from build123d import *

# Parameters (mm, degrees)
F0_R     = 23
F0_R_2   = 20
F1_DEPTH = 20
F2_R     = 23
F3_DEPTH = 5
F4_R     = 1
F5_R     = 1


with BuildPart() as f1:
    # F0 (on Top) → F1 (new body)
    with BuildSketch(Plane.XY):
        Circle(F0_R)
        Circle(F0_R_2, mode=Mode.SUBTRACT)
    extrude(amount=F1_DEPTH)

    # F2 (on face) → F3 (join)
    with BuildSketch(Plane.XY.offset(20)):
        Circle(F2_R)
    extrude(amount=F3_DEPTH)

    # F4
    f4_edges = [f1.edges().sort_by_distance(p)[0] for p in [
        (-20, 0, 0),
    ]]
    fillet(f4_edges, radius=F4_R)

    # F5
    f5_edges = [f1.edges().sort_by_distance(p)[0] for p in [
        (-23, 0, 0),
    ]]
    fillet(f5_edges, radius=F5_R)


solid = f1.part
Here's how the part is built. I have some questions about the finished solid (model axes, mm). Round coordinates to 2 decimals unless told otherwise and drop trailing zeros. Order: outer loops, then holes, each group sorted by start corner. A loop starts at its lowest first (then second) coordinate and runs counter-clockwise, first axis right, second up. Notation, with made-up numbers: M 25,46.5 L 64,46.5 A13 ccw 64,66.5 Z; hole C 1.25,11 d10. An arc over 180 degrees is marked long. Return JSON: item names as keys, results as strings. Group by question number.
1. If we section it at C-C on z = 2.75: List the corners of the cut face in (x, y) for me.
2. If we section it at D-D on z = 21.25: List the corners of the cut face in (x, y) for me, then the cut area to 3 significant figures.
3. I'm going to push flat-ended pins straight in: pin 1 Ø3 at (x, z) = (10.5, 3.5) entering from -Y; pin 2 Ø1.5 at (y, z) = (8, 3.5) entering from +X; pin 3 Ø1.5 at (y, z) = (1, 17) entering from -X. Where does each tip first touch, or does it pass through?
4. Please list where these lines run through material, in increasing order: probe 1 along Y at (x, z) = (0, 5); probe 2 along Z at (x, y) = (15.5, -11); probe 3 along Y at (x, z) = (-13, 18.5).
5. If we mould it in two halves opening along Y, with no side actions, what happens to faces 1 (the face through (-4.336, -19.524, 10.367)), 2 (the face through (0, 0, 25)), 3 (the face through (-2.994, 22.804, 12.832))? For each: pulls with the +Y half, pulls with the -Y half, needs draft (parallel to the pull), parting line crosses it, or undercut.
6. If we section it at A-A on y = 0: List the corners of the cut face in (x, z) for me, then the cut area to 3 significant figures.
Reply:
{
 "1": {"outline": "C 0,0 d46; hole C 0,0 d40"},
 "2": {"outline": "C 0,0 d46", "area": "1,660 mm^2"},
 "3": {"pin 1": "y = -21.17", "pin 2": "x = 21.83", "pin 3": "x = -23"},
 "4": {"probe 1": "-23 to -20, 20 to 23", "probe 2": "20 to 25", "probe 3": "-18.97 to -15.2, 15.2 to 18.97"},
 "5": {"face 1": "undercut", "face 2": "needs draft", "face 3": "parting line crosses it"},
 "6": {"outline": "M -23,1 A1 ccw -22,0 L -21,0 A1 ccw -20,1 L -20,20 L 20,20 L 20,1 A1 ccw 21,0 L 22,0 A1 ccw 23,1 L 23,25 L -23,25 Z", "area": "349 mm^2"}
}
